Could you check a few things on this model? Use its own coordinates, in mm. Round coordinates to 2 decimals unless told otherwise and drop trailing zeros. Write each loop counter-clockwise with the first axis right and the second up, starting at its lowest first coordinate (ties: lowest second). Pieces come first, ordered by that corner, then holes. Notation, with made-up numbers: (85, 71.5) - (133, 71.5) arc R24 ccw to (133, 109.5) - close; hole circle Ø3 at (82.25, 77). An arc over 180 degrees is marked (long way). Put each result on its own line as item: value.
from build123d import *

# Parameters (mm, degrees)
SKETCH2_R                    = 7.9375
SKETCH2_R_2                  = 3.7465
BOSS_EXTRUDE1_DEPTH          = 204.47
FILLET1_R                    = 3.81
CIRPATTERN1_COUNT            = 4
FILLET1_OF_CIRPATTERN1_R     = 3.81
SKETCH3_R                    = 8.636
CUT_EXTRUDE1_DEPTH           = 12.7
CIRPATTERN2_COUNT            = 4
FILLET2_R                    = 2.54
MIRROR1_COPY_1_SKETCH_R      = 8.636
MIRROR1_COPY_1_DEPTH         = 12.7
MIRROR1_COPY_2_SKETCH_R      = 8.636
MIRROR1_COPY_2_DEPTH         = 12.7
MIRROR1_COPY_3_SKETCH_R      = 8.636
MIRROR1_COPY_3_DEPTH         = 12.7
FILLET3_R                    = 2.54
F_5_16_CLEARANCE_HOLE1_D     = 8.4328
F_5_16_CLEARANCE_HOLE1_DEPTH = 54.864
F_5_16_CLEARANCE_HOLE1_TIP   = 2.533468714
F_6_CLEARANCE_HOLE1_D        = 3.7973
F_6_CLEARANCE_HOLE1_DEPTH    = 54.864
F_6_CLEARANCE_HOLE1_TIP      = 1.140824014
CUT_EXTRUDE2_START           = -204.47
SKETCH9_R                    = 52.832
CUT_EXTRUDE2_DEPTH           = 95.504


with BuildPart() as part:
    # Sketch1 → Revolve1 (revolve)
    with BuildSketch(Plane.XY, mode=Mode.PRIVATE) as revolve1_sk:
        Polygon((44.45, 0), (44.45, 204.47), (50.6984, 204.47), (50.6984, 108.966), (52.832, 108.966), (52.832, 95.504), (50.6984, 95.504), (50.6984, 0), align=None)
    revolve(revolve1_sk.sketch.rotate(Axis((0, 138.931800571, 0), (0, -1, 0)), 180), axis=Axis((0, 138.931800571, 0), (0, -1, 0)))

    # Sketch2 → Boss-Extrude1 (add)
    with BuildSketch(Plane(origin=(0, 204.47, 0), x_dir=(1, 0, 0), z_dir=(0, 1, 0))):
        with Locations((0, 40.7035)):
            Circle(SKETCH2_R)
        with Locations(Location((0, 40.7035, 0), (0, 0, 180))):
            Circle(SKETCH2_R_2, mode=Mode.SUBTRACT)
    boss_extrude1 = extrude(amount=-BOSS_EXTRUDE1_DEPTH)

    # Fillet1
    fillet1_edges = [part.edges().sort_by_distance(p)[0] for p in [
        (-7.287865551, 102.235, -43.848483619),
        (7.287865551, 102.235, -43.848483619),
    ]]
    fillet(fillet1_edges, radius=FILLET1_R)

    # CirPattern1: Boss-Extrude1 ×4 about axis
    cirpattern1_axis = Axis((0, 0, 0), (0, 1, 0))
    for i in range(1, CIRPATTERN1_COUNT):
        add(boss_extrude1.rotate(cirpattern1_axis, i * 360 / CIRPATTERN1_COUNT))

    # Fillet1 of CirPattern1
    fillet1_of_cirpattern1_edges = [part.edges().sort_by_distance(p)[0] for p in [
        (-43.848483619, 102.235, 7.287865551),
        (-43.848483619, 102.235, -7.287865551),
        (7.287865551, 102.235, 43.848483619),
        (-7.287865551, 102.235, 43.848483619),
        (43.848483619, 102.235, -7.287865551),
        (43.848483619, 102.235, 7.287865551),
    ]]
    fillet(fillet1_of_cirpattern1_edges, radius=FILLET1_OF_CIRPATTERN1_R)

    # Sketch3 → Cut-Extrude1 (cut)
    with BuildSketch(Plane(origin=(0, 204.47, 0), x_dir=(1, 0, 0), z_dir=(0, 1, 0))):
        with Locations((0, 40.7035)):
            Circle(SKETCH3_R)
    cut_extrude1 = extrude(amount=-CUT_EXTRUDE1_DEPTH, mode=Mode.SUBTRACT)

    # CirPattern2: Cut-Extrude1 ×4 about axis
    cirpattern2_axis = Axis((0, 0, 0), (0, 1, 0))
    for i in range(1, CIRPATTERN2_COUNT):
        add(cut_extrude1.rotate(cirpattern2_axis, i * 360 / CIRPATTERN2_COUNT), mode=Mode.SUBTRACT)

    # Fillet2
    fillet2_edges = [part.edges().sort_by_distance(p)[0] for p in [
        (-8.61576795, 198.12, -41.294294914),
        (8.61576795, 198.12, -41.294294914),
        (-41.294294914, 198.12, 8.61576795),
        (8.61576795, 198.12, 41.294294914),
        (41.294294914, 198.12, -8.61576795),
        (41.294294914, 198.12, 8.61576795),
        (-8.61576795, 198.12, 41.294294914),
        (-41.294294914, 198.12, -8.61576795),
    ]]
    fillet(fillet2_edges, radius=FILLET2_R)

    # Mirror1: Cut-Extrude1 across plane
    add(cut_extrude1.mirror(Plane.ZX.offset(102.235)), mode=Mode.SUBTRACT)

    # Mirror1 copy 1 sketch → Mirror1 copy 1 (cut)
    with BuildSketch(Plane(origin=(0, 0, 0), x_dir=(0, 0, -1), z_dir=(0, -1, 0))):
        with Locations((0, -40.7035)):
            Circle(MIRROR1_COPY_1_SKETCH_R)
    extrude(amount=-MIRROR1_COPY_1_DEPTH, mode=Mode.SUBTRACT)

    # Mirror1 copy 2 sketch → Mirror1 copy 2 (cut)
    with BuildSketch(Plane(origin=(0, 0, 0), x_dir=(-1, 0, 0), z_dir=(0, -1, 0))):
        with Locations((0, -40.7035)):
            Circle(MIRROR1_COPY_2_SKETCH_R)
    extrude(amount=-MIRROR1_COPY_2_DEPTH, mode=Mode.SUBTRACT)

    # Mirror1 copy 3 sketch → Mirror1 copy 3 (cut)
    with BuildSketch(Plane(origin=(0, 0, 0), x_dir=(0, 0, 1), z_dir=(0, -1, 0))):
        with Locations((0, -40.7035)):
            Circle(MIRROR1_COPY_3_SKETCH_R)
    extrude(amount=-MIRROR1_COPY_3_DEPTH, mode=Mode.SUBTRACT)

    # Fillet3
    fillet3_edges = [part.edges().sort_by_distance(p)[0] for p in [
        (-41.294294914, 6.35, 8.61576795),
        (8.61576795, 6.35, 41.294294914),
        (41.294294914, 6.35, -8.61576795),
        (-8.61576795, 6.35, -41.294294914),
        (8.61576795, 6.35, -41.294294914),
        (41.294294914, 6.35, 8.61576795),
        (-8.61576795, 6.35, 41.294294914),
        (-41.294294914, 6.35, -8.61576795),
    ]]
    fillet(fillet3_edges, radius=FILLET3_R)

    # 5/16 Clearance Hole1
    with Locations(Plane(origin=(37.357865464, 0, 37.357865464), x_dir=(0, 1, 0), z_dir=(0.7071067811865488, 0, 0.7071067811865464))):
        with Locations((102.235, -9.525), (102.235, 9.525)):
            Hole(F_5_16_CLEARANCE_HOLE1_D / 2, depth=F_5_16_CLEARANCE_HOLE1_DEPTH)
            with Locations((0, 0, -(F_5_16_CLEARANCE_HOLE1_DEPTH + F_5_16_CLEARANCE_HOLE1_TIP / 2))):  # 118° drill point
                Cone(0, F_5_16_CLEARANCE_HOLE1_D / 2, F_5_16_CLEARANCE_HOLE1_TIP, mode=Mode.SUBTRACT)

    # #6 Clearance Hole1
    with Locations(Plane(origin=(37.357865464, 0, -37.357865464), x_dir=(0, 1, 0), z_dir=(0.7071067811865438, 0, -0.7071067811865512))):
        with Locations((102.235, 0)):
            Hole(F_6_CLEARANCE_HOLE1_D / 2, depth=F_6_CLEARANCE_HOLE1_DEPTH)
            with Locations((0, 0, -(F_6_CLEARANCE_HOLE1_DEPTH + F_6_CLEARANCE_HOLE1_TIP / 2))):  # 118° drill point
                Cone(0, F_6_CLEARANCE_HOLE1_D / 2, F_6_CLEARANCE_HOLE1_TIP, mode=Mode.SUBTRACT)

    # Sketch9 → Cut-Extrude2 (cut)
    with BuildSketch(Plane(origin=(0, 204.47, 0), x_dir=(1, 0, 0), z_dir=(0, 1, 0)).offset(CUT_EXTRUDE2_START)):
        with Locations(Location((0, 0, 0), (0, 0, 180))):
            Circle(SKETCH9_R)
    extrude(amount=CUT_EXTRUDE2_DEPTH, mode=Mode.SUBTRACT)

    # Sketch11 → Cut-Revolve2 (revolve, cut)
    with BuildSketch(Plane.XY):
        Polygon((48.641, 95.504), (0, 95.504), (0, 204.47), (50.6984, 204.47), (50.6984, 108.966), (48.641, 108.966), align=None)
    revolve(axis=Axis((0, 95.504, 0), (0, 1, 0)), mode=Mode.SUBTRACT)


solid = part.part
(1) If we mould it in two halves opening along Z, with no side actions, what happens to faces 1 (the face through (-50.39, 102.14, -15.87)), 2 (the face through (-15, 95.504, -47)), 3 (the face through (27.423, 98.213, 42.684)), 4 (the face through (44.43, 100.29, 25.67))? For each: pulls with the +Z half, pulls with the -Z half, needs draft (parallel to the pull), parting line crosses it, or undercut.
Values found:
face 1: parting line crosses it
face 2: needs draft
face 3: undercut
face 4: undercut
(2) Imagine slicing it at A-A, the plane x = 0. List the corners of the cut face in (y, z) for me, then the cut area to 3 significant figures.
Values found:
outline: (95.5, -52.83) - (108.97, -52.83) - (108.97, -48.64) - (95.5, -48.64) - close; (95.5, 48.64) - (108.97, 48.64) - (108.97, 52.83) - (95.5, 52.83) - close
area: 113 mm^2
(3) I'm going to push flat-ended pins straight in: pin 1 (4 mm diameter, centred on y = 102, z = 6.5, fed in from -X); pin 2 (1.5 mm diameter, centred on y = 99, z = 12, fed in from -X); pin 3 (5 mm diameter, centred on x = -23.5, y = 100, fed in from +Z). Where does each tip first touch, or does it pass through?
Values found:
pin 1: stops at x = -52.64
pin 2: stops at x = -51.62
pin 3: stops at z = 48.48
(4) Imagine slicing it at B-B, the plane z = 0. List the corners of the cut face in (x, y) for me, then the cut area to 3 significant figures.
Values found:
outline: (-52.83, 95.5) - (-48.64, 95.5) - (-48.64, 108.97) - (-52.83, 108.97) - close; (48.64, 95.5) - (52.83, 95.5) - (52.83, 108.97) - (48.64, 108.97) - close
area: 113 mm^2
(5) Please list where these lines run through material, in increasing order: probe 1 along X at (y, z) = (100, 0); probe 2 along X at (y, z) = (102, 38.5). Write a range as from..to.
Values found:
probe 1: x = -52.83..-48.64, 48.64..52.83
probe 2: x = -36.18..-29.73, 30.98..36.18
